Study the drawing (mm; zero at the part's minimum x, y, z) and answer. Coordinates: 2 decimals unless noted, no trailing zeros. Loops run counter-clockwise (first coordinate to the right, second up) from the corner with the lowest first, then second, coordinate; pieces in that order, holes last. Notation, with made-up numbers: (79.25, 9.5) -> (99.25, 9.5) arc R7 cw to (99.25, 22.5) -> close; hole circle Ø2 at (84, 33). An arc over 180 degrees is marked (long way). Answer in a Markdown table with one row per item.
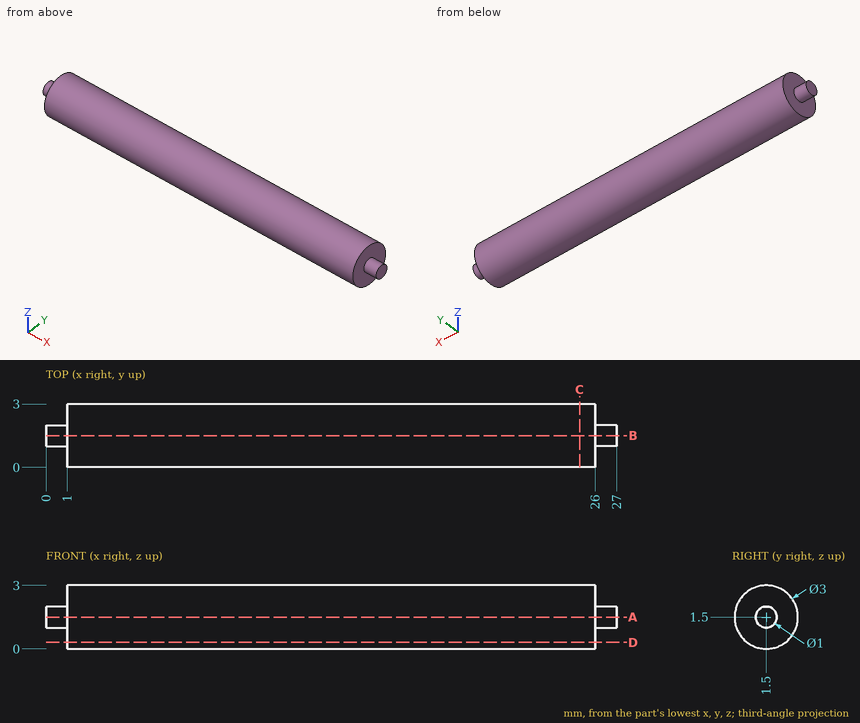
1. A cutting plane is placed at A-A on z = 1.5. Give the vertices of the cut face in (x, y), and give its area (3 significant figures).
A:
| item | result |
|---|---|
| outline | (0, 1) -> (1, 1) -> (1, 0) -> (26, 0) -> (26, 1) -> (27, 1) -> (27, 2) -> (26, 2) -> (26, 3) -> (1, 3) -> (1, 2) -> (0, 2) -> close |
| area | 77.0 mm2 |
2. Given pin 1 Ø1.5 at (x, y) = (21.5, 0.5) entering from -Z, flat-ended and moving along its own axis, determine where the tip first touches the part or whether it passes through.
A:
| item | result |
|---|---|
| pin 1 | stops at z = 0.02 |
3. A cutting plane is placed at C-C on x = 25.25. Give the vertices of the cut face in (y, z).
A:
| item | result |
|---|---|
| outline | circle Ø3 at (1.5, 1.5) |
4. Find the intervals of material crossed by probe 1 along X at (y, z) = (1.1, 0.9); probe 2 along Z at (x, y) = (9.25, 1.6); probe 3 along Z at (x, y) = (4.5, 2.15), in increasing order.
A:
| item | result |
|---|---|
| probe 1 | x = 1 to 26 |
| probe 2 | z = 0 to 3 |
| probe 3 | z = 0.15 to 2.85 |
5. A cutting plane is placed at D-D on z = 0.3. Give the vertices of the cut face in (x, y), and give its area (3 significant figures).
A:
| item | result |
|---|---|
| outline | (1, 0.6) -> (26, 0.6) -> (26, 2.4) -> (1, 2.4) -> close |
| area | 45.0 mm2 |
